from build123d import *

# Parameters (mm, degrees)
SKETCH1_R           = 55
BOSS_EXTRUDE2_DEPTH = 20
SKETCH2_R           = 51
CUT_EXTRUDE1_DEPTH  = 17
SKETCH10_R          = 1.5
BOSS_EXTRUDE3_DEPTH = 10
SKETCH10_3_W        = 7
SKETCH10_3_H        = 7
CUT_EXTRUDE4_DEPTH  = 10
FILLET1_R           = 3


with BuildPart() as part:
    # Sketch1 → Boss-Extrude2 (new body)
    with BuildSketch(Plane.XY):
        with Locations((328.389379834, 629.271631436)):
            Circle(SKETCH1_R)
    extrude(amount=BOSS_EXTRUDE2_DEPTH)

    # Sketch2 → Cut-Extrude1 (cut)
    with BuildSketch(Plane(origin=(0, 0, 0), x_dir=(-1, 0, 0), z_dir=(0, 0, -1))):
        with Locations((-328.628637891, 629.384320649)):
            Circle(SKETCH2_R)
    extrude(amount=-CUT_EXTRUDE1_DEPTH, mode=Mode.SUBTRACT)

    # Sketch10 → Boss-Extrude3 (add)
    with BuildSketch(Plane(origin=(0, 0, 17), x_dir=(-1, 0, 0), z_dir=(0, 0, -1))):
        with Locations((-374.389379834, 627.076422512)):
            Circle(SKETCH10_R)
        with Locations((-282.389379834, 627.076422512)):
            Circle(SKETCH10_R)
    extrude(amount=BOSS_EXTRUDE3_DEPTH)

    # Sketch10<3> → Cut-Extrude4 (cut)
    with BuildSketch(Plane(origin=(0, 0, 17), x_dir=(-1, 0, 0), z_dir=(0, 0, -1))):
        with Locations((-328.389379834, 627.076422512)):
            Rectangle(SKETCH10_3_W, SKETCH10_3_H)
        with Locations((-310.889379834, 627.076422512)):
            Rectangle(SKETCH10_3_W, SKETCH10_3_H)
        with Locations((-293.389379834, 627.076422512)):
            Rectangle(SKETCH10_3_W, SKETCH10_3_H)
        with Locations((-345.889379834, 627.076422512)):
            Rectangle(SKETCH10_3_W, SKETCH10_3_H)
        with Locations((-363.389379834, 627.076422512)):
            Rectangle(SKETCH10_3_W, SKETCH10_3_H)
    extrude(amount=-CUT_EXTRUDE4_DEPTH, mode=Mode.SUBTRACT)

    # Fillet1
    fillet1_edges = [part.edges().sort_by_distance(p)[0] for p in [
        (273.389379834, 629.271631436, 20),
    ]]
    fillet(fillet1_edges, radius=FILLET1_R)


solid = part.part
Input: part model. Units: mm. Frame: model coordinates. A direction names the side the tool comes from. Give positions to 0.01 mm unless a question says otherwise; leave off trailing zeros. Order: outer loops, then holes, each group sorted by start corner. A loop starts at its lowest first (then second) coordinate and runs counter-clockwise, first axis right, second up. Notation, with made-up numbers: (35, 8.25) - (74, 8.25) arc R20 ccw to (74, 35.25) - close; hole circle Ø7 at (81.25, -16.75). An arc over 180 degrees is marked (long way). Answer as a JSON object with one key per item and string values. Group by question number.
Q1. Set-up query: faces 4 (the face through (282, 627, 7)), 5 (the face through (359.889, 627, 18)), 6 (the face through (303.7, 584.7, 0)). Return all of +Z, -Z, +X, -X, +Y, -Y with unobstructed straight access to the full face (end or side cutting, diameter ignored); none if empty.
Q2. Line query: probe 1 along Z at (x, y) = (353.5, 587); probe 2 along X at (y, z) = (619, 1.5); probe 3 along X at (y, z) = (666, 6.75). Output: solid intervals per line, ascending.
Q3. First-contact query: pin 1 Ø10 at (x, y) = (348.5, 616.5) entering from -Z; pin 2 Ø3.5 at (x, z) = (363.5, 19) entering from +Y; pin 3 Ø1.5 at (x, z) = (346, 18.5) entering from +Y. Flat tips, straight axial feed; report the tip coordinate or a pass-through.
Q4. Cut plane B-B, the plane z = 3. Output: boundary loops of the cut face in (x, y).
Q5. Cut plane A-A, the plane z = 15.5. Output: boundary loops of the cut face in (x, y), then the cut area to 3 significant figures.
Q6. Mould query, pull axis X, two halves, no side actions, for faces 1 (the face through (346, 630.576, 18)), 2 (the face through (339, 630, 20)), 3 (the face through (316.47, 575.58, 8.38)). Classes: pulls with the +X half, pulls with the -X half, needs draft (parallel to the pull), parting line crosses it, or undercut.
Results:
{
 "1": {"face 4": "-Z", "face 5": "+Z, -Z", "face 6": "-Z, +X, -X, +Y, -Y"},
 "2": {"probe 1": "17 to 20", "probe 2": "274.36 to 278.7, 378.56 to 382.42", "probe 3": "287.45 to 293.13, 364.13 to 369.33"},
 "3": {"pin 1": "z = 17", "pin 2": "y = 672.54", "pin 3": "y = 681.38"},
 "4": {"outline": "circle Ø110 at (328.39, 629.27); hole circle Ø102 at (328.63, 629.38)"},
 "5": {"outline": "circle Ø110 at (328.39, 629.27); circle Ø3 at (282.39, 627.08); circle Ø3 at (374.39, 627.08); hole circle Ø102 at (328.63, 629.38)", "area": "1,350 mm^2"},
 "6": {"face 1": "undercut", "face 2": "needs draft", "face 3": "parting line crosses it"}
}
